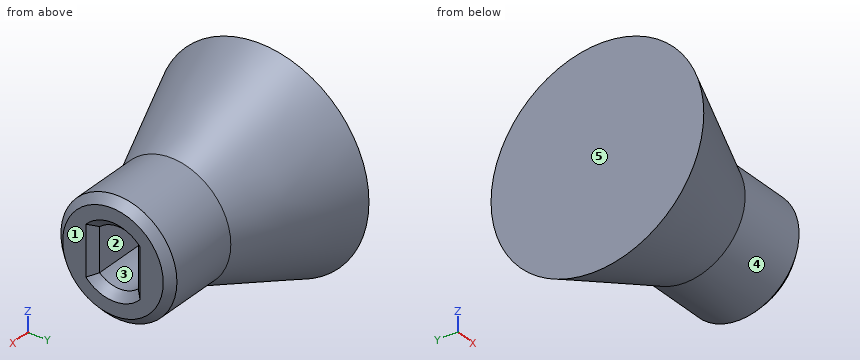
from build123d import *

# Parameters (mm, degrees)
CUT_EXTRUDE1_DEPTH = 8
CHAMFER1_SIZE      = 0.8


with BuildPart() as part:
    # Sketch2 → Revolve1 (revolve)
    with BuildSketch(Plane.XY):
        Polygon((0, 0), (0, 11), (12, 6), (20, 6), (20, 0), align=None)
    revolve(axis=Axis((20, 0, 0), (-1, 0, 0)))

    # Sketch3 → Cut-Extrude1 (cut)
    with BuildSketch(Plane(origin=(20, 0, 0), x_dir=(0, 0, -1), z_dir=(1, 0, 0))):
        with BuildLine():
            Line((-2.236067977, 2), (2.236067977, 2))
            ThreePointArc((2.236067977, 2), (3, 0), (2.236067977, -2))
            Line((2.236067977, -2), (-2.236067977, -2))
            ThreePointArc((-2.236067977, -2), (-3, 0), (-2.236067977, 2))
        make_face()
    extrude(amount=-CUT_EXTRUDE1_DEPTH, mode=Mode.SUBTRACT)

    # Chamfer1
    chamfer1_edges = [part.edges().sort_by_distance(p)[0] for p in [
        (20, 0, 3),
        (20, -2, 0),
        (20, 0, -3),
        (20, 2, 0),
        (20, -6, 0),
    ]]
    chamfer(chamfer1_edges, length=CHAMFER1_SIZE)


solid = part.part
CAD build for the part. Positions are in the model's coordinates, mm. Face numbers are marked on the shaded views. A direction names the side the tool comes from. Give positions to 0.01 mm unless a question says otherwise; leave off trailing zeros. Loops run counter-clockwise (first coordinate to the right, second up) from the corner with the lowest first, then second, coordinate; pieces in that order, holes last. Notation, with made-up numbers: M 83,-7.75 L 108,-7.75 A21 ccw 108,12.25 Z; hole C 0.5,85 d6. An arc over 180 degrees is marked long. One line per question, with ' | ' between items. Start each with the question number.
1. Probe L1, parallel to Z at x = 7, y = 7.5 (3 decimals); L2, parallel to Y at x = 18.25, z = 1.5; L3, parallel to Z at x = 10.25, y = 5.75. List the from-to ranges inside material, lowest first. Write a range as from..to.
2. Saw through at C-C on y = 0. Give the cut face in (x, z), plus the area to 3 significant figures.
3. Flat gauge pins, fed straight in: pin 1 (3 mm diameter, centred on x = 16.5, y = -3, fed in from -Z); pin 2 (3.5 mm diameter, centred on x = 15.5, z = 0, fed in from -Y); pin 3 (1 mm diameter, centred on y = 1, z = 8, fed in from +X). Where does each tip first touch, or does it go through?
4. Two-plate mould, pull along Y, no slides. Class the marked faces 3, 4 and 5: pulls with the +Y half, pulls with the -Y half, needs draft (parallel to the pull), parting line crosses it, or undercut.
5. Saw through at B-B on z = 0. Give the cut face in (x, y), plus the area to 3 significant figures.
6. Saw through at D-D on x = 9. Give the cut face in (y, z).
7. Saw through at A-A on x = 13.75. Give the cut face in (y, z), plus the area to 3 significant figures.
8. 3-axis set-ups, long thin cutter, end or side, ignore diameter. For the marked faces 1 and 2: which of +Z, -Z, +X, -X, +Y, -Y reach the whole face in a straight line?
Result sheet:
1) L1: z = -3.015..3.015 | L2: y = -5.81..-2, 2..5.81 | L3: z = -3.5..3.5
2) outline: M 0,-11 L 12,-6 L 19.2,-6 L 20,-5.2 L 20,-3.8 L 19.2,-3 L 12,-3 L 12,3 L 19.2,3 L 20,3.8 L 20,5.2 L 19.2,6 L 12,6 L 0,11 Z | area: 251 mm^2
3) pin 1: stops at z = -5.81 | pin 2: stops at y = -6 | pin 3: stops at x = 8.25
4) face 3: undercut | face 4: parting line crosses it | face 5: needs draft
5) outline: M 0,-11 L 12,-6 L 19.2,-6 L 20,-5.2 L 20,-2.8 L 19.2,-2 L 12,-2 L 12,2 L 19.2,2 L 20,2.8 L 20,5.2 L 19.2,6 L 12,6 L 0,11 Z | area: 267 mm^2
6) outline: C 0,0 d14.5
7) outline: C 0,0 d12; hole M -2,-2.24 A3 ccw 2,-2.24 L 2,2.24 A3 ccw -2,2.24 Z | area: 91.0 mm^2
8) face 1: +Z, -Z, +X, +Y, -Y | face 2: +X
